```python
from build123d import *

# Parameters (mm, degrees)
SKETCH1_R               = 9
MAIN_BODY_DEPTH         = 15
SKETCH4_R               = 6.4
BOSS_EXTRUDE3_DEPTH     = 2.5
SKETCH5_R               = 3.9
BOSS_EXTRUDE4_DEPTH     = 7
SKETCH9_R               = 2
ARM_ATTTACH_DEPTH       = 3
SKETCH11_W              = 18
SKETCH11_H              = 12
CUT_EXTRUDE1_DEPTH      = 5
SKETCH13_R              = 2
ARM_ATTACH_DEPTH        = 3
CUT_EXTRUDE5_DEPTH      = 12
SKETCH14_W              = 6
SKETCH14_H              = 8
BLADE_HOLE_DEPTH        = 12
SKETCH21_W              = 15
SKETCH21_H              = 12
FACE_CUT_DEPTH          = 10
SKETCH23_R              = 9
SKETCH23_R_2            = 7
CUT_EXTRUDE8_DEPTH      = 4
SKETCH24_R              = 1.75
SCREW_HOLE_DEPTH        = 15
SKETCH26_R              = 1.65
CUT_EXTRUDE9_DEPTH      = 16
CUT_EXTRUDE9_DEPTH_BACK = 10.5


with BuildPart() as part:
    # Sketch1 → main body (new body)
    with BuildSketch(Plane(origin=(0, 0, 0), x_dir=(1, 0, 0), z_dir=(0, 1, 0))):
        Circle(SKETCH1_R)
    extrude(amount=MAIN_BODY_DEPTH)

    # Sketch4 → Boss-Extrude3 (add)
    with BuildSketch(Plane.XZ):
        Circle(SKETCH4_R)
    extrude(amount=BOSS_EXTRUDE3_DEPTH)

    # Sketch5 → Boss-Extrude4 (add)
    with BuildSketch(Plane.XZ.offset(2.5)):
        Circle(SKETCH5_R)
    extrude(amount=BOSS_EXTRUDE4_DEPTH)

    # Sketch9 → arm atttach (add)
    with BuildSketch(Plane.XZ):
        with BuildLine():
            Line((0, 9), (0, 13))
            ThreePointArc((0, 13), (4.5, 17.5), (9, 13))
            Line((9, 13), (9, 0))
            ThreePointArc((9, 0), (6.363961031, 6.363961031), (0, 9))
        make_face()
        with Locations((4.5, 13)):
            Circle(SKETCH9_R, mode=Mode.SUBTRACT)
    extrude(amount=-ARM_ATTTACH_DEPTH)

    # Sketch11 → Cut-Extrude1 (cut)
    with BuildSketch(Plane(origin=(5, 0, 0), x_dir=(0, 0, -1), z_dir=(1, 0, 0))):
        with Locations((0, 9)):
            Rectangle(SKETCH11_W, SKETCH11_H)
    extrude(amount=CUT_EXTRUDE1_DEPTH, mode=Mode.SUBTRACT)

    # Sketch13 → arm attach (add)
    with BuildSketch(Plane(origin=(0, 8, 0), x_dir=(1, 0, 0), z_dir=(0, 1, 0))):
        with BuildLine():
            Line((0, -13), (0, -9))
            ThreePointArc((0, -9), (2.61248608, -8.61248608), (5, -7.483314774))
            Line((5, -7.483314774), (5, -3.50923953))
            Line((5, -3.50923953), (9, -7.42923953))
            Line((9, -7.42923953), (9, -13))
            ThreePointArc((9, -13), (4.5, -17.5), (0, -13))
        make_face()
        with Locations((4.5, -13)):
            Circle(SKETCH13_R, mode=Mode.SUBTRACT)
    extrude(amount=ARM_ATTACH_DEPTH)

    # Sketch19 → Cut-Extrude5 (cut)
    with BuildSketch(Plane(origin=(0, 15, 0), x_dir=(1, 0, 0), z_dir=(0, 1, 0))):
        with BuildLine():
            Line((0, -7), (0, -9))
            ThreePointArc((0, -9), (-3.939351121, 8.092064801), (7.083885455, -5.551447276))
            Line((7.083885455, -5.551447276), (5.644138479, -4.14049524))
            ThreePointArc((5.644138479, -4.14049524), (-3.163584464, 6.244336101), (0, -7))
        make_face()
    extrude(amount=-CUT_EXTRUDE5_DEPTH, mode=Mode.SUBTRACT)

    # Sketch14 → blade hole (cut)
    with BuildSketch(Plane(origin=(0, 15, 0), x_dir=(1, 0, 0), z_dir=(0, 1, 0))):
        Rectangle(SKETCH14_W, SKETCH14_H)
    extrude(amount=-BLADE_HOLE_DEPTH, mode=Mode.SUBTRACT)

    # Sketch21 → face cut (cut)
    with BuildSketch(Plane.ZY.offset(5)):
        with Locations((0, 9)):
            Rectangle(SKETCH21_W, SKETCH21_H)
    extrude(amount=FACE_CUT_DEPTH, mode=Mode.SUBTRACT)

    # Sketch23 → Cut-Extrude8 (cut)
    with BuildSketch(Plane(origin=(0, 15, 0), x_dir=(1, 0, 0), z_dir=(0, 1, 0))):
        Circle(SKETCH23_R)
        Circle(SKETCH23_R_2, mode=Mode.SUBTRACT)
    extrude(amount=-CUT_EXTRUDE8_DEPTH, mode=Mode.SUBTRACT)

    # Sketch24 → screw hole (cut, symmetric)
    with BuildSketch(Plane.ZY.offset(5)):
        with Locations((0, 9)):
            Circle(SKETCH24_R)
    extrude(amount=SCREW_HOLE_DEPTH, both=True, mode=Mode.SUBTRACT)

    # Sketch26 → Cut-Extrude9 (cut, two sides)
    with BuildSketch(Plane(origin=(0, 0, 0), x_dir=(1, 0, 0), z_dir=(0, 1, 0))) as cut_extrude9_sk:
        Circle(SKETCH26_R)
    extrude(amount=CUT_EXTRUDE9_DEPTH, mode=Mode.SUBTRACT)
    extrude(cut_extrude9_sk.sketch, amount=-CUT_EXTRUDE9_DEPTH_BACK, mode=Mode.SUBTRACT)


solid = part.part
```
Verification items for the finished model (mm, model axes). A direction names the side the tool comes from. Coordinates: 2 decimals unless noted, no trailing zeros. Order: outer loops, then holes, each group sorted by start corner. A loop starts at its lowest first (then second) coordinate and runs counter-clockwise, first axis right, second up. Notation, with made-up numbers: (-1.75, -32) -> (22.25, -32) arc R24 cw to (22.25, 6) -> close; hole circle Ø6 at (29.5, 56). An arc over 180 degrees is marked (long way). Answer as CSV lines item,"result". Start each with the question number.
1) Cross-section at B-B, the plane y = 9. Record the boundary of the cut face in (x, z), then the cut area to 3 significant figures.
2) Cross-section at C-C, the plane x = 4.5. Record the boundary of the cut face in (y, z), then the cut area to 3 significant figures.
3) Cross-section at D-D, the plane y = 2. Record the boundary of the cut face in (x, z), then the cut area to 3 significant figures.
4) Cross-section at A-A, the plane z = 9.75. Record the boundary of the cut face in (x, y), then the cut area to 3 significant figures.
5) Release check for a two-part mould opening along Y. For faces 4 (the face through (9, 1, 7)), 5 (the face through (2, 0, 7)), 6 (the face through (5, 10.4, 1.4)) record: released by +Y, released by -Y, zero draft, split by the parting line, or undercut.
6) Gauge pin test, flat ends, axial feed: pin 1 Ø10 at (x, z) = (6.5, 13) entering from +Y; pin 2 Ø4.5 at (y, z) = (9, 0) entering from -X; pin 3 Ø6 at (x, z) = (2, 7.5) entering from -Y. Record the tip position at first contact, or that the pin passes through.
7) Material ranges on L1, parallel to Y at x = 4, z = 9; L2, parallel to X at y = 3.25, z = 2.25; L3, parallel to Y at x = -2.75, z = -1, recorded low to high. Write a range as [from, to].
8) Set-up check for faces 1 (the face through (5, 8, 10)), 2 (the face through (-2.87, -5.95, 2.64)), 3 (the face through (0, 3, -2)): record each of +Z, -Z, +X, -X, +Y, -Y from which the full face is reachable in a straight line by a thin tool's end or side.
Conclusion:
1,outline,"(-5, -4.9) arc R7 ccw to (5, -4.9) -> (5, -1.75) -> (3, -1.75) -> (3, -4) -> (-3, -4) -> (-3, -1.75) -> (-5, -1.75) -> close; (-5, 1.75) -> (-3, 1.75) -> (-3, 4) -> (3, 4) -> (3, 1.75) -> (5, 1.75) -> (5, 3.51) -> (9, 7.43) -> (9, 13) arc R4.5 ccw to (0, 13) -> (0, 7) arc R7 ccw to (-5, 4.9) -> close; hole circle Ø4 at (4.5, 13)"
1,area,"148 mm²"
2,outline,"(-2.5, -4.55) -> (0, -4.55) -> (0, -7.79) -> (3, -7.79) -> (3, -5.36) -> (15, -5.36) -> (15, 5.36) -> (11, 5.36) -> (11, 11) -> (8, 11) -> (8, 7.79) -> (3, 7.79) -> (3, 11) -> (0, 11) -> (0, 4.55) -> (-2.5, 4.55) -> close; (0, 15) -> (3, 15) -> (3, 17.5) -> (0, 17.5) -> close; (8, 15) -> (11, 15) -> (11, 17.5) -> (8, 17.5) -> close; hole circle Ø3.5 at (9, 0)"
2,area,"242 mm²"
3,outline,"(0, 9) arc R9 ccw (long way) to (9, 0) -> (9, 13) arc R4.5 ccw to (0, 13) -> close; hole circle Ø3.3 at (0, 0); hole circle Ø4 at (4.5, 13)"
3,area,"319 mm²"
4,outline,"(0, 0) -> (9, 0) -> (9, 3) -> (0, 3) -> close; (0, 8) -> (9, 8) -> (9, 11) -> (0, 11) -> close"
4,area,"54.0 mm²"
5,face 4,"zero draft"
5,face 5,"released by -Y"
5,face 6,"undercut"
6,pin 1,"stops at y = 11"
6,pin 2,"stops at x = -5"
6,pin 3,"stops at y = -2.5"
7,L1,"y = [0, 3], [8, 11]"
7,L2,"x = [-5, -3], [3, 5]"
7,L3,"y = [-9.5, 3]"
8,face 1,"+Z, +X"
8,face 2,"-Y"
8,face 3,"+Y"
